```python
from build123d import *

# Parameters (mm, degrees)
SKETCH1_R                = 25
BOSS_EXTRUDE1_DEPTH      = 25
SKETCH2_R                = 48
BOSS_EXTRUDE2_DEPTH      = 10
SKETCH3_R                = 30.78576119
BOSS_EXTRUDE3_DEPTH      = 41
BOSS_EXTRUDE4_DEPTH      = 113
BOSS_EXTRUDE4_DEPTH_BACK = 31
SKETCH5_W                = 12
SKETCH5_H                = 50
BOSS_EXTRUDE5_DEPTH      = 122
BOSS_EXTRUDE5_DEPTH_BACK = 21
SKETCH6_W                = 12
SKETCH6_H                = 50
SKETCH7_R                = 3
CUT_EXTRUDE1_DEPTH       = 25
BOSS_EXTRUDE6_DEPTH      = 128
BOSS_EXTRUDE6_DEPTH_BACK = 16
SKETCH9_W                = 53.159298554
SKETCH9_H                = 15
SKETCH8_R                = 7.5
CUT_EXTRUDE2_DEPTH       = 10
SKETCH10_R               = 4
CUT_EXTRUDE3_DEPTH       = 72
SKETCH11_R               = 4
CUT_EXTRUDE4_DEPTH       = 72


with BuildPart() as part:
    # Sketch1 → Boss-Extrude1 (new body)
    with BuildSketch(Plane.XY):
        Circle(SKETCH1_R)
    extrude(amount=BOSS_EXTRUDE1_DEPTH)

    # Sketch2 → Boss-Extrude2 (add)
    with BuildSketch(Plane.XY.offset(25)):
        Circle(SKETCH2_R)
    extrude(amount=BOSS_EXTRUDE2_DEPTH)

    # Sketch3 → Boss-Extrude3 (add)
    with BuildSketch(Plane.XY.offset(35)):
        Circle(SKETCH3_R)
    extrude(amount=BOSS_EXTRUDE3_DEPTH)

    # Sketch5 → Boss-Extrude4 (add, two sides: drawn at the far end of the back side and taken through both)
    with BuildSketch(Plane(origin=(-25.371352033, -17.437247146, 0), x_dir=(0, 0, 1), z_dir=(-0.8241261886220168, -0.5664062369248312, 0)).offset(-BOSS_EXTRUDE4_DEPTH_BACK)):
        with Locations((51, -0.21423881)):
            Rectangle(SKETCH5_W, SKETCH5_H)
    extrude(amount=BOSS_EXTRUDE4_DEPTH + BOSS_EXTRUDE4_DEPTH_BACK)

    # Sketch6 → Boss-Extrude5 (add, two sides: drawn at the far end of the back side and taken through both)
    with BuildSketch(Plane(origin=(25.371352033, -17.437247146, 0), x_dir=(0, 0, -1), z_dir=(0.8241261886220168, -0.5664062369248313, 0)).offset(-BOSS_EXTRUDE5_DEPTH_BACK)):
        with Locations((-51, -0.21423881)):
            Rectangle(SKETCH6_W, SKETCH6_H)
    extrude(amount=BOSS_EXTRUDE5_DEPTH + BOSS_EXTRUDE5_DEPTH_BACK)

    # Sketch7 → Cut-Extrude1 (cut)
    with BuildSketch(Plane(origin=(0, 0, 0), x_dir=(-1, 0, 0), z_dir=(0, 0, -1))):
        Circle(SKETCH7_R)
    extrude(amount=-CUT_EXTRUDE1_DEPTH, mode=Mode.SUBTRACT)

    # Sketch9 → Boss-Extrude6 (add, two sides: drawn at the far end of the back side and taken through both)
    with BuildSketch(Plane(origin=(0, 30.78576119, 0), x_dir=(1, 0, 0), z_dir=(0, 1, 0)).offset(-BOSS_EXTRUDE6_DEPTH_BACK)):
        with Locations((0.01957738, -52.5)):
            Rectangle(SKETCH9_W, SKETCH9_H)
    extrude(amount=BOSS_EXTRUDE6_DEPTH + BOSS_EXTRUDE6_DEPTH_BACK)

    # Sketch8 → Cut-Extrude2 (cut)
    with BuildSketch(Plane.XY.offset(76)):
        with Locations((-13, 0)):
            Circle(SKETCH8_R)
        with Locations((13, 0)):
            Circle(SKETCH8_R)
        with Locations((0, 13)):
            Circle(SKETCH8_R)
        with Locations((0, -13)):
            Circle(SKETCH8_R)
    extrude(amount=-CUT_EXTRUDE2_DEPTH, mode=Mode.SUBTRACT)

    # Sketch10 → Cut-Extrude3 (cut)
    with BuildSketch(Plane.XY.offset(57)):
        with Locations((-104.853188395, -57.155978452)):
            Circle(SKETCH10_R)
        with Locations((-90.693032472, -77.759133168)):
            Circle(SKETCH10_R)
    cut_extrude3 = extrude(amount=-CUT_EXTRUDE3_DEPTH, mode=Mode.SUBTRACT)

    # Mirror1: Cut-Extrude3 across plane
    add(cut_extrude3.mirror(Plane.ZY), mode=Mode.SUBTRACT)

    # Sketch11 → Cut-Extrude4 (cut)
    with BuildSketch(Plane.XY.offset(60)):
        with Locations((0.01957738, 133.78576119)):
            Circle(SKETCH11_R)
    extrude(amount=-CUT_EXTRUDE4_DEPTH, mode=Mode.SUBTRACT)


solid = part.part
```
For this review, take the finished solid that the model builds, in its own axes (mm). A direction names the side the tool comes from. Give positions to 0.01 mm unless a question says otherwise; leave off trailing zeros. Write each loop counter-clockwise with the first axis right and the second up, starting at its lowest first coordinate (ties: lowest second). Pieces come first, ordered by that corner, then holes.
Item 1: Take a section at B-B (z = 31). Give the boundary of the cut face in (x, y).
Item 2: Insertion check: P1, Ø12, axis at y = -3.5, z = 15.5, coming from the +X side; P2, Ø10, axis at y = -51.5, z = 42.5, coming from the +X side; P3, Ø4.5, axis at x = 3, y = 16.5, coming from the +Z side. Each pin has a flat end and moves straight along its axis. Give the tip position at first contact, or say it passes through.
Item 3: Take a section at C-C (y = -13). Give the boundary of the cut face in (x, z), and give its area (3 significant figures).
Item 4: Take a section at D-D (x = 13). Give the boundary of the cut face in (y, z), and give its area (3 significant figures).
Item 5: Machinability: for faces 5 (the face through (-26.56, 86, 53)), 6 (the face through (13, 0, 66)), 7 (the face through (-51.518, -66.003, 50.916)), 8 (the face through (21, -21, 25)), which of the approach directions +Z, -Z, +X, -X, +Y, -Y give a long, thin tool a straight path to every point of the face, cutting with its end or side? Answer none if there is none.
Item 6: Take a section at A-A (x = 43.5). Give the boundary of the cut face in (y, z), and give its area (3 significant figures).
Item 7: The part is to be moulded in two halves that separate along Y. For faces 1 (the face through (-20.493, 0.33, 71.07)), 2 (the face through (5.507, 0.33, 71.07)), 3 (the face through (-118.575, -81.329, 50.916)), 4 (the face through (69, -48, 45)), say which applies: +Y half, -Y half, draft (parallel to the pull), parting line (faces both ways), or undercut.
Item 8: Wall thickness on probe 1 along Y at (x, z) = (0, 71); probe 2 along Y at (x, z) = (0, 18); probe 3 along Z at (x, y) = (-66, -35.5): over which ranges is each line inside the solid? List them lowest first.
Established:
1. outline: circle Ø96 at (0, 0)
2. P1: stops at x = 25
2. P2: stops at x = 124.99
2. P3: stops at z = 66
3. outline: (-62.67, 45) - (-27.91, 45) - (-27.91, 35) - (-46.21, 35) - (-46.21, 25) - (-21.35, 25) - (-21.35, 0) - (21.35, 0) - (21.35, 25) - (46.21, 25) - (46.21, 35) - (27.91, 35) - (27.91, 45) - (62.67, 45) - (62.67, 57) - (27.91, 57) - (27.91, 76) - (7.5, 76) - (7.5, 66) - (-7.5, 66) - (-7.5, 76) - (-27.91, 76) - (-27.91, 57) - (-62.67, 57) - close
3. area: 4,960 mm2
4. outline: (-46.21, 25) - (-21.35, 25) - (-21.35, 0) - (21.35, 0) - (21.35, 25) - (46.21, 25) - (46.21, 35) - (27.91, 35) - (27.91, 45) - (158.79, 45) - (158.79, 60) - (27.91, 60) - (27.91, 76) - (7.5, 76) - (7.5, 66) - (-7.5, 66) - (-7.5, 76) - (-27.91, 76) - (-27.91, 57) - (-39.53, 57) - (-39.53, 45) - (-27.91, 45) - (-27.91, 35) - (-46.21, 35) - close
4. area: 6,230 mm2
5. face 5: +Z, -X, +Y
5. face 6: +Z
5. face 7: +Z, -Y
5. face 8: -Z
6. outline: (-60.49, 45) - (0.18, 45) - (0.18, 57) - (-60.49, 57) - close; (-20.29, 25) - (20.29, 25) - (20.29, 35) - (-20.29, 35) - close
6. area: 1,130 mm2
7. face 1: undercut
7. face 2: undercut
7. face 3: -Y half
7. face 4: draft
8. probe 1: y = -30.79 to -20.5, -5.5 to 5.5, 20.5 to 30.79
8. probe 2: y = -25 to -3, 3 to 25
8. probe 3: z = 45 to 57
